Input: part model. Units: mm. Frame: model coordinates. Face numbers are marked on the shaded views. A direction names the side the tool comes from. Give positions to 0.01 mm unless a question says otherwise; leave off trailing zeros. Loops run counter-clockwise (first coordinate to the right, second up) from the corner with the lowest first, then second, coordinate; pieces in that order, holes last. Notation, with made-up numbers: (26, 89.5) -> (65, 89.5) arc R18 ccw to (65, 118.5) -> close; hole circle Ø6 at (88, 46). An arc over 180 degrees is marked (long way). Use CSV: the item, a comma, the result in double quotes.
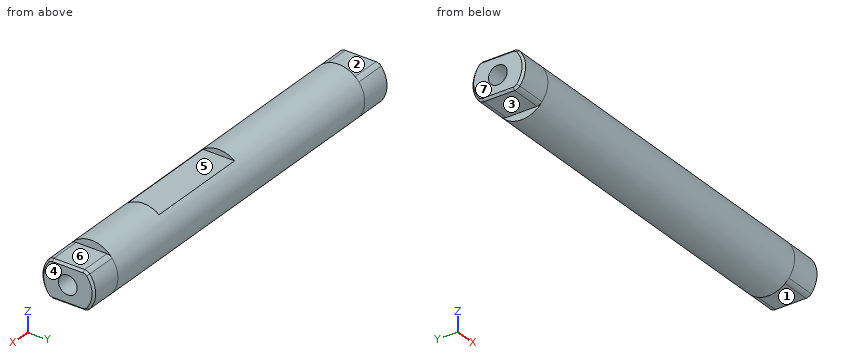
```python
from build123d import *

# Parameters (mm, degrees)
SKETCH1_R                = 3.175
BOSS_EXTRUDE1_DEPTH      = 20.7645
BOSS_EXTRUDE2_START      = 4.0005
BOSS_EXTRUDE2_DEPTH      = 4.0005
FILLET1_R                = 0.79375
CHAMFER1_SIZE            = 0.254
FILLET1_OF_MIRROR2_R     = 0.79375
CHAMFER1_OF_MIRROR2_SIZE = 0.254
SKETCH5_W                = 12.7
SKETCH5_H                = 6.35
CUT_EXTRUDE1_DEPTH       = 0.635


with BuildPart() as part:
    # Sketch1 → Boss-Extrude1 (new, symmetric)
    with BuildSketch(Plane(origin=(0, 0, 0), x_dir=(0, 0, -1), z_dir=(1, 0, 0))):
        Circle(SKETCH1_R)
    extrude(amount=BOSS_EXTRUDE1_DEPTH, both=True)

    # Sketch2 → Boss-Extrude2 (add)
    with BuildSketch(Plane(origin=(20.7645, 0, 0), x_dir=(0, 0, -1), z_dir=(1, 0, 0)).offset(BOSS_EXTRUDE2_START)):
        with BuildLine():
            Line((-2.286, 2.20336765), (-2.286, -2.20336765))
            ThreePointArc((-2.286, -2.20336765), (0, -3.175), (2.286, -2.20336765))
            Line((2.286, -2.20336765), (2.286, 2.20336765))
            ThreePointArc((2.286, 2.20336765), (0, 3.175), (-2.286, 2.20336765))
        make_face()
    boss_extrude2 = extrude(amount=-BOSS_EXTRUDE2_DEPTH)

    # Fillet1
    # the kernel refuses this fillet: 0.79375 mm, written as the material it takes off along each edge
    with BuildSketch(Plane(origin=(25.768693051, 2.20336765, -2.286), x_dir=(0, 0.6746831627986616, 0.7381074649642793), z_dir=(-1, 0, 0)), Plane(origin=(25.768693051, -2.20336765, 2.286), x_dir=(0, -0.6746831627986605, -0.7381074649642803), z_dir=(-1, 0, 0))) as fillet1_piece_1:
        with BuildLine():
            CenterArc((0.351292568, -0.792161955), FILLET1_R, 86.375070371, 51.195378821)
            Line((-0.234580233, -0.256632195), (0, 0))
            ThreePointArc((0, 0), (0.20073861, 0.006352179), (0.40147722, 0))
        make_face()
    extrude(amount=5.004193051, mode=Mode.SUBTRACT)
    with BuildSketch(Plane(origin=(25.768693051, -2.20336765, -2.286), x_dir=(0, -0.6746831627986618, 0.738107464964279), z_dir=(-1, 0, 0)), Plane(origin=(25.768693051, 2.20336765, 2.286), x_dir=(0, 0.6746831627986606, -0.73810746496428), z_dir=(-1, 0, 0))) as fillet1_piece_2:
        with BuildLine():
            CenterArc((0.351292568, 0.792161955), FILLET1_R, 222.429550808, 51.195378821)
            Line((-0.234580233, 0.256632195), (0, 0))
            ThreePointArc((0, 0), (0.20073861, -0.006352179), (0.40147722, 0))
        make_face()
    extrude(amount=5.004193051, mode=Mode.SUBTRACT)

    # Sketch3 → #4-40 Tapped Hole1 (revolve, cut)
    with BuildSketch(Plane(origin=(24.765, 0, 0), x_dir=(0, 0, -1), z_dir=(0, 1, 0))):
        Polygon((0, 0), (0, 8.299152758), (1.1303, 7.62), (1.1303, 0), align=None)
    f_4_40_tapped_hole1 = revolve(axis=Axis((31.115, 0, 0), (-1, 0, 0)), mode=Mode.SUBTRACT)

    # Chamfer1
    chamfer1_edges = [part.edges().sort_by_distance(p)[0] for p in [
        (24.765, 0, -2.286),
        (24.765, 3.175, 0),
        (24.765, -3.175, 0),
        (24.765, 0, 2.286),
        (24.765, 2.198617373, 2.208093398),
        (24.765, -2.198617373, 2.208093398),
        (24.765, 2.198617373, -2.208093398),
        (24.765, -2.198617373, -2.208093398),
    ]]
    chamfer(chamfer1_edges, length=CHAMFER1_SIZE)

    # Mirror2: Boss-Extrude2, #4-40 Tapped Hole1 across plane
    add(boss_extrude2.mirror(Plane(origin=(0, 0, 0), x_dir=(0, 0, 1), z_dir=(1, 0, 0))))
    add(f_4_40_tapped_hole1.mirror(Plane(origin=(0, 0, 0), x_dir=(0, 0, 1), z_dir=(1, 0, 0))), mode=Mode.SUBTRACT)

    # Fillet1 of Mirror2
    # the kernel refuses this fillet: 0.79375 mm, written as the material it takes off along each edge
    with BuildSketch(Plane(origin=(-25.768693051, 2.20336765, -2.286), x_dir=(0, 0.6746831627986613, 0.7381074649642795), z_dir=(1, 0, 0)), Plane(origin=(-25.768693051, -2.20336765, 2.286), x_dir=(0, -0.67468316279866, -0.7381074649642806), z_dir=(1, 0, 0))) as fillet1_of_mirror2_piece_1:
        with BuildLine():
            CenterArc((0.351292568, 0.792161955), FILLET1_OF_MIRROR2_R, 222.429550808, 51.195378821)
            Line((-0.234580233, 0.256632195), (0, 0))
            ThreePointArc((0, 0), (0.20073861, -0.006352179), (0.40147722, 0))
        make_face()
    extrude(amount=5.004193051, mode=Mode.SUBTRACT)
    with BuildSketch(Plane(origin=(-25.768693051, -2.20336765, -2.286), x_dir=(0, -0.6746831627986595, 0.738107464964281), z_dir=(1, 0, 0)), Plane(origin=(-25.768693051, 2.20336765, 2.286), x_dir=(0, 0.674683162798661, -0.7381074649642797), z_dir=(1, 0, 0))) as fillet1_of_mirror2_piece_2:
        with BuildLine():
            CenterArc((0.351292568, -0.792161955), FILLET1_OF_MIRROR2_R, 86.375070371, 51.195378821)
            Line((-0.234580233, -0.256632195), (0, 0))
            ThreePointArc((0, 0), (0.20073861, 0.006352179), (0.40147722, 0))
        make_face()
    extrude(amount=5.004193051, mode=Mode.SUBTRACT)

    # Chamfer1 of Mirror2
    chamfer1_of_mirror2_edges = [part.edges().sort_by_distance(p)[0] for p in [
        (-24.765, 0, -2.286),
        (-24.765, 3.175, 0),
        (-24.765, -3.175, 0),
        (-24.765, 0, 2.286),
        (-24.765, 2.198617373, 2.208093398),
        (-24.765, -2.198617373, 2.208093398),
        (-24.765, 2.198617373, -2.208093398),
        (-24.765, -2.198617373, -2.208093398),
    ]]
    chamfer(chamfer1_of_mirror2_edges, length=CHAMFER1_OF_MIRROR2_SIZE)

    # Sketch5 → Cut-Extrude1 (cut)
    with BuildSketch(Plane.XY.offset(3.175)):
        with Locations((5.715, 0)):
            Rectangle(SKETCH5_W, SKETCH5_H)
    extrude(amount=-CUT_EXTRUDE1_DEPTH, mode=Mode.SUBTRACT)


solid = part.part
```
1) Reachability of the marked faces 1, 2 and 3 from +Z, -Z, +X, -X, +Y, -Y: full face, straight path, thin tool, end or side. Return the list, or none.
From the geometry:
face 1,"-Z, +X, +Y, -Y"
face 2,"+Z, -X, +Y, -Y"
face 3,"-Z, -X, +Y, -Y"
2) Ray query, line 1 (Z direction, x = -21.75, y = 0); line 2 (Z direction, x = -19.75, y = 0) (3 decimals); line 3 (Z direction, x = -5, y = -1.25). Return the intervals inside material, ascending.
From the geometry:
line 1,"z = -2.29 to -1.13, 1.13 to 2.29"
line 2,"z = -3.175 to -1.13, 1.13 to 3.175"
line 3,"z = -2.92 to 2.92"
3) Section query A-A (x = 20). Return loops of the section in (y, z) (3 decimals).
From the geometry:
outline,"circle Ø6.35 at (0, 0); hole circle Ø2.261 at (0, 0)"
4) Contact query for flat-ended pins moving along their axis: pin 1 (3 mm diameter, centred on x = -11, y = -2, fed in from -Z); pin 2 (1.1 mm diameter, centred on x = 23, y = -0.5, fed in from +Z); pin 3 (1.4 mm diameter, centred on y = 0, z = 0, fed in from -X). Output: stop coordinate, or through.
From the geometry:
pin 1,"stops at z = -3.14"
pin 2,"stops at z = 2.29"
pin 3,"stops at x = -16.89"
5) Mould query, pull axis X, two halves, no side actions, for the marked faces 4, 5, 6 and 7. Classes: pulls with the +X half, pulls with the -X half, needs draft (parallel to the pull), parting line crosses it, or undercut.
From the geometry:
face 4,"pulls with the +X half"
face 5,"undercut"
face 6,"needs draft"
face 7,"pulls with the -X half"
